CAD build for the part. Positions are in the model's coordinates, mm. Face numbers are marked on the shaded views. A direction names the side the tool comes from. Round coordinates to 2 decimals unless told otherwise and drop trailing zeros. Write each loop counter-clockwise with the first axis right and the second up, starting at its lowest first coordinate (ties: lowest second). Pieces come first, ordered by that corner, then holes. Notation, with made-up numbers: (23, 11) - (60, 11) arc R21 ccw to (60, 36) - close; hole circle Ø1 at (-18, -20). An arc over 180 degrees is marked (long way). Answer in a Markdown table with one row per item.
```python
from build123d import *

# Parameters (mm, degrees)
F1_DEPTH = 9.525
F2_W     = 12.7
F2_H     = 9.525
F3_DEPTH = 6.35
F5_DEPTH = 4.7625
F7_R     = 1.5875
F6_R     = 1.5875
F8_DEPTH = 25.4


# Not quite as in the source:
# - a feature names something its author has since deleted; it is built from what else it names


with BuildPart() as f1:
    # F0 (on Top) → F1 (new body)
    with BuildSketch(Plane.XY):
        with BuildLine():
            ThreePointArc((0, 9.525), (-4.7625, 4.7625), (0, 0))
            Line((0, 0), (25.4, 0))
            ThreePointArc((25.4, 0), (30.1625, 4.7625), (25.4, 9.525))
            Line((25.4, 9.525), (0, 9.525))
        make_face()
    extrude(amount=F1_DEPTH)

    # F2 (on face) → F3 (cut)
    with BuildSketch(Plane(origin=(0, 0, 0), x_dir=(1, 0, 0), z_dir=(0, 0, -1))):
        with Locations((12.7, -4.7625)):
            Rectangle(F2_W, F2_H)
    extrude(amount=-F3_DEPTH, mode=Mode.SUBTRACT)

    # F4 (on face) → F5 (cut)
    with BuildSketch(Plane.XY.offset(9.525)):
        with BuildLine():
            Line((4.7625, 9.525), (0, 9.525))
            ThreePointArc((0, 9.525), (-4.7625, 4.7625), (0, 0))
            Line((0, 0), (4.7625, 0))
            Line((4.7625, 0), (4.7625, 9.525))
        make_face()
        with BuildLine():
            Line((25.4, 9.525), (20.6375, 9.525))
            Line((20.6375, 9.525), (20.6375, 0))
            Line((20.6375, 0), (25.4, 0))
            ThreePointArc((25.4, 0), (30.1625, 4.7625), (25.4, 9.525))
        make_face()
    extrude(amount=-F5_DEPTH, mode=Mode.SUBTRACT)

    # F7 (on face) + F6 (on face) → F8 (cut)
    with BuildSketch(Plane.XY.offset(4.7625)):
        with Locations((0, 4.7625)):
            Circle(F7_R)
    with BuildSketch(Plane.XY.offset(4.7625)):
        with Locations((25.4, 4.7625)):
            Circle(F6_R)
    extrude(amount=-F8_DEPTH, mode=Mode.SUBTRACT)


solid = f1.part
```
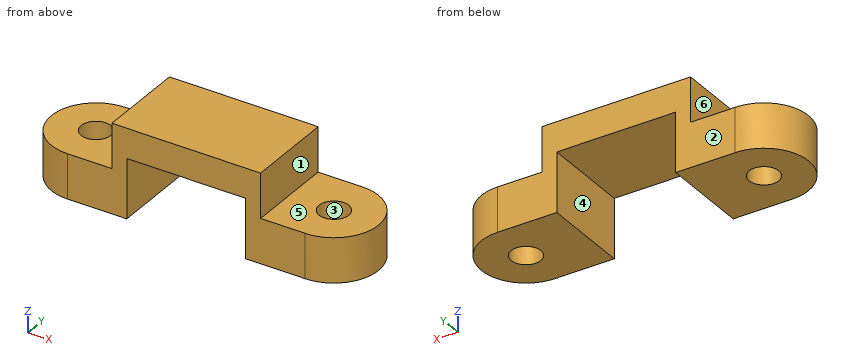
Q1. Saw through at A-A on z = 4. Count the separate pieces of the cut face and the enclosed holes in it, then the cut area to 3 significant figures.
Computed:
| item | result |
|---|---|
| separate pieces | 2 |
| enclosed holes | 2 |
| area | 176 mm2 |
Q2. Saw through at B-B on x = 1. List the corners of the cut face in (y, z) (1 decimal).
Computed:
| item | result |
|---|---|
| outline | (0, 0) - (3.5, 0) - (3.5, 4.8) - (0, 4.8) - close; (6, 0) - (9.5, 0) - (9.5, 4.8) - (6, 4.8) - close |
Q3. Drill centre lines: line 1 (X direction, y = 4.75, z = 2.75); line 2 (Y direction, x = 25.4, z = 3.75) (3 decimals); line 3 (Z direction, x = 27, y = 5.75). Where is each one in solid material? Low to high.
Computed:
| item | result |
|---|---|
| line 1 | x = -4.76 to -1.59, 1.59 to 6.35, 19.05 to 23.81, 26.99 to 30.16 |
| line 2 | y = 0 to 3.175, 6.35 to 9.525 |
| line 3 | z = 0 to 4.76 |
Q4. Pull direction Y, two halves, no side cores. Call the marked faces 1, 2 and 3: released by +Y, released by -Y, zero draft, split by the parting line, or undercut.
Computed:
| item | result |
|---|---|
| face 1 | zero draft |
| face 2 | released by +Y |
| face 3 | undercut |
Q5. 3-axis set-ups, long thin cutter, end or side, ignore diameter. For the marked faces 4, 5 and 6: which of +Z, -Z, +X, -X, +Y, -Y reach the whole face in a straight line?
Computed:
| item | result |
|---|---|
| face 4 | -Z, +Y, -Y |
| face 5 | +Z, +X, +Y, -Y |
| face 6 | +Z, -X, +Y, -Y |
Q6. Flat gauge pins, fed straight in: pin 1 (5 mm diameter, centred on x = 11.5, y = 2.5, fed in from -Z); pin 2 (1.9 mm diameter, centred on x = 25.4, y = 4.76, fed in from -Z); pin 3 (5 mm diameter, centred on x = -1, y = 3.5, fed in from +Z); pin 4 (4 mm diameter, centred on y = 6.5, z = 7.5, fed in from -X). Where does each tip first touch, or does it go through?
Computed:
| item | result |
|---|---|
| pin 1 | stops at z = 6.35 |
| pin 2 | passes through |
| pin 3 | stops at z = 4.76 |
| pin 4 | stops at x = 4.76 |
